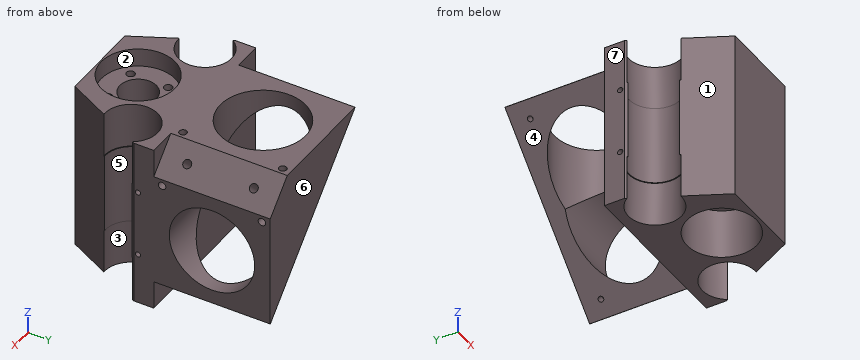
```python
from build123d import *

# Parameters (mm, degrees)
BOSS_EXTRUDE1_DEPTH        = 51
CUT_EXTRUDE1_REACH         = 53
SKETCH2_R                  = 7.75
CUT_EXTRUDE2_REACH         = 53
SKETCH6_R                  = 5.5
M3_TAPPED_HOLE2_D          = 2.5
M3_TAPPED_HOLE2_DEPTH      = 11.5
M3_TAPPED_HOLE2_TIP        = 0.751075774
SKETCH13_R                 = 10.5
CUT_EXTRUDE5_DEPTH         = 15
BOSS_EXTRUDE2_DEPTH        = 35
CUT_EXTRUDE6_REACH         = 53
SKETCH24_R                 = 12.8397
CUT_EXTRUDE7_REACH         = 53
SKETCH25_R                 = 12.8397
M2_TAPPED_HOLE1_D          = 1.6
M2_TAPPED_HOLE1_DEPTH      = 3.2
M2_TAPPED_HOLE1_TIP        = 0.480688495
M3_TAPPED_HOLE4_D          = 2.5
M3_TAPPED_HOLE4_DEPTH      = 7.5
M3_TAPPED_HOLE4_TIP        = 0.751075774
M2_TAPPED_HOLE2_AT_2_COUNT = 2
M2_TAPPED_HOLE2_AT_2_PITCH = 20
SKETCH38_R                 = 11.1
CUT_EXTRUDE8_DEPTH         = 5.5
SKETCH39_R                 = 8
CUT_EXTRUDE9_DEPTH         = 13.5
SKETCH41_R                 = 8
CUT_EXTRUDE10_DEPTH        = 13.5
F_4_40_TAPPED_HOLE1_D      = 2.2606
F_4_40_TAPPED_HOLE1_DEPTH  = 7.59
F_4_40_TAPPED_HOLE1_TIP    = 0.679152758
F_4_40_TAPPED_HOLE2_D      = 2.2606
F_4_40_TAPPED_HOLE2_DEPTH  = 7.6
F_4_40_TAPPED_HOLE2_TIP    = 0.679152758


with BuildPart() as part:
    # Sketch1 → Boss-Extrude1 (new body)
    with BuildSketch(Plane.XY):
        Polygon((-25.5, 0), (25.5, 0), (25.5, -6), (12.5, -31.5), (-12.5, -31.5), (-25.5, -6), align=None)
    extrude(amount=BOSS_EXTRUDE1_DEPTH)

    # Sketch2 → Cut-Extrude1 (cut, up to next)
    with BuildSketch(Plane.XY.offset(51), mode=Mode.PRIVATE) as cut_extrude1_sk1:
        with Locations((-18.5, -11)):
            Circle(SKETCH2_R)
    cut_extrude1_tool1 = extrude(cut_extrude1_sk1.sketch, amount=-CUT_EXTRUDE1_REACH, mode=Mode.PRIVATE) & part.part
    add(cut_extrude1_tool1.solids().sort_by_distance((-18.5, -11, 51))[0], mode=Mode.SUBTRACT)
    # Sketch2 → Cut-Extrude1 (cut, up to next)
    with BuildSketch(Plane.XY.offset(51), mode=Mode.PRIVATE) as cut_extrude1_sk2:
        with Locations((18.5, -11)):
            Circle(SKETCH2_R)
    cut_extrude1_tool2 = extrude(cut_extrude1_sk2.sketch, amount=-CUT_EXTRUDE1_REACH, mode=Mode.PRIVATE) & part.part
    add(cut_extrude1_tool2.solids().sort_by_distance((18.5, -11, 51))[0], mode=Mode.SUBTRACT)

    # Sketch6 → Cut-Extrude2 (cut, up to next)
    with BuildSketch(Plane.XY.offset(51), mode=Mode.PRIVATE) as cut_extrude2_sk1:
        with Locations((0, -20)):
            Circle(SKETCH6_R)
    cut_extrude2_tool1 = extrude(cut_extrude2_sk1.sketch, amount=-CUT_EXTRUDE2_REACH, mode=Mode.PRIVATE) & part.part
    add(cut_extrude2_tool1.solids().sort_by_distance((0, -20, 51))[0], mode=Mode.SUBTRACT)

    # M3 Tapped Hole2
    with Locations(Plane.XY.offset(51)):
        with Locations((-5.656854249, -14.343145751), (5.656854249, -25.656854249), (5.656854249, -14.343145751), (-5.656854249, -25.656854249)):
            Hole(M3_TAPPED_HOLE2_D / 2, depth=M3_TAPPED_HOLE2_DEPTH)
            with Locations((0, 0, -(M3_TAPPED_HOLE2_DEPTH + M3_TAPPED_HOLE2_TIP / 2))):  # 118° drill point
                Cone(0, M3_TAPPED_HOLE2_D / 2, M3_TAPPED_HOLE2_TIP, mode=Mode.SUBTRACT)

    # Sketch13 → Cut-Extrude5 (cut)
    with BuildSketch(Plane(origin=(0, 0, 0), x_dir=(-1, 0, 0), z_dir=(0, 0, -1))):
        with Locations((0, -20)):
            Circle(SKETCH13_R)
    extrude(amount=-CUT_EXTRUDE5_DEPTH, mode=Mode.SUBTRACT)

    # Sketch22 → Boss-Extrude2 (add)
    with BuildSketch(Plane(origin=(0, 0, 0), x_dir=(1, 0, 0), z_dir=(0, 1, 0))):
        Polygon((-16.970562748, -50.955844123), (-16.970562748, -51), (16.970562748, -51), (25.5, -42.470562748), (25.5, -8.529437252), (25.455844123, -8.529437252), align=None)
    extrude(amount=BOSS_EXTRUDE2_DEPTH)

    # Sketch24 → Cut-Extrude6 (cut, up to next)
    with BuildSketch(Plane.XY.offset(51), mode=Mode.PRIVATE) as cut_extrude6_sk1:
        with Locations((0, 17.5)):
            Circle(SKETCH24_R)
    cut_extrude6_tool1 = extrude(cut_extrude6_sk1.sketch, amount=-CUT_EXTRUDE6_REACH, mode=Mode.PRIVATE) & part.part
    add(cut_extrude6_tool1.solids().sort_by_distance((0, 17.5, 51))[0], mode=Mode.SUBTRACT)

    # Sketch25 → Cut-Extrude7 (cut, up to next)
    with BuildSketch(Plane(origin=(25.5, 0, 0), x_dir=(0, 0, -1), z_dir=(1, 0, 0)), mode=Mode.PRIVATE) as cut_extrude7_sk1:
        with Locations((-25.5, 17.5)):
            Circle(SKETCH25_R)
    cut_extrude7_tool1 = extrude(cut_extrude7_sk1.sketch, amount=-CUT_EXTRUDE7_REACH, mode=Mode.PRIVATE) & part.part
    add(cut_extrude7_tool1.solids().sort_by_distance((25.5, 17.5, 25.5))[0], mode=Mode.SUBTRACT)

    # M2 Tapped Hole1
    with Locations(Plane(origin=(16.992640687, 0, 16.992640687), x_dir=(-0.707106781, 0, 0.707106781), z_dir=(-0.707106781, 0, -0.707106781))):
        with Locations((43.03122292, 29.5), (-6.96877708, 5.5), (-6.96877708, 29.5), (43.03122292, 5.5)):
            Hole(M2_TAPPED_HOLE1_D / 2, depth=M2_TAPPED_HOLE1_DEPTH)
            with Locations((0, 0, -(M2_TAPPED_HOLE1_DEPTH + M2_TAPPED_HOLE1_TIP / 2))):  # 118° drill point
                Cone(0, M2_TAPPED_HOLE1_D / 2, M2_TAPPED_HOLE1_TIP, mode=Mode.SUBTRACT)

    # M3 Tapped Hole4
    with Locations(Plane(origin=(33.985281374, 0, 33.985281374), x_dir=(0.707106781, 0, -0.707106781), z_dir=(0.707106781, 0, 0.707106781))):
        with Locations((-18.03122292, 27.5), (-18.03122292, 7.5)):
            Hole(M3_TAPPED_HOLE4_D / 2, depth=M3_TAPPED_HOLE4_DEPTH)
            with Locations((0, 0, -(M3_TAPPED_HOLE4_DEPTH + M3_TAPPED_HOLE4_TIP / 2))):  # 118° drill point
                Cone(0, M3_TAPPED_HOLE4_D / 2, M3_TAPPED_HOLE4_TIP, mode=Mode.SUBTRACT)

    # Sketch36 → M2 Tapped Hole2 (revolve, cut)
    with BuildSketch(Plane(origin=(25.5, -4.75, 35.5), x_dir=(0, 0, -1), z_dir=(0, 1, 0))):
        Polygon((0, 0), (0, 7.680688495), (0.8, 7.2), (0.8, 0), align=None)
    m2_tapped_hole2 = revolve(axis=Axis((31.85, -4.75, 35.5), (-1, 0, 0)), mode=Mode.SUBTRACT)

    # M2 Tapped Hole2 at 2: M2 Tapped Hole2 ×2
    with Locations(*[(0, 0, -i * M2_TAPPED_HOLE2_AT_2_PITCH) for i in range(1, M2_TAPPED_HOLE2_AT_2_COUNT)]):
        add(m2_tapped_hole2, mode=Mode.SUBTRACT)

    # Mirror1: M2 Tapped Hole2 across plane
    add(m2_tapped_hole2.mirror(Plane(origin=(0, 0, 0), x_dir=(0, 0, 1), z_dir=(1, 0, 0))), mode=Mode.SUBTRACT)

    # Mirror1 copy 1 sketch → Mirror1 copy 1 (revolve, cut)
    with BuildSketch(Plane(origin=(-25.5, -4.75, 15.5), x_dir=(0, 0, -1), z_dir=(0, 1, 0))):
        Polygon((0, 0), (0, -7.680688495), (0.8, -7.2), (0.8, 0), align=None)
    revolve(axis=Axis((-31.85, -4.75, 15.5), (-1, 0, 0)), mode=Mode.SUBTRACT)

    # Sketch38 → Cut-Extrude8 (cut)
    with BuildSketch(Plane.XY.offset(51)):
        with Locations((0, -20)):
            Circle(SKETCH38_R)
    extrude(amount=-CUT_EXTRUDE8_DEPTH, mode=Mode.SUBTRACT)

    # Sketch39 → Cut-Extrude9 (cut)
    with BuildSketch(Plane(origin=(0, 0, 0), x_dir=(-1, 0, 0), z_dir=(0, 0, -1))):
        with Locations((18.5, -11)):
            Circle(SKETCH39_R)
        with Locations((-18.5, -11)):
            Circle(SKETCH39_R)
    extrude(amount=-CUT_EXTRUDE9_DEPTH, mode=Mode.SUBTRACT)

    # Sketch41 → Cut-Extrude10 (cut)
    with BuildSketch(Plane.XY.offset(51)):
        with Locations((18.5, -11)):
            Circle(SKETCH41_R)
        with Locations((-18.5, -11)):
            Circle(SKETCH41_R)
    extrude(amount=-CUT_EXTRUDE10_DEPTH, mode=Mode.SUBTRACT)

    # #4-40 Tapped Hole1
    with Locations(Plane(origin=(25.5, 0, 0), x_dir=(0, 0, -1), z_dir=(1, 0, 0))):
        with Locations((-40.5, 32.5), (-40.5, 2.5)):
            Hole(F_4_40_TAPPED_HOLE1_D / 2, depth=F_4_40_TAPPED_HOLE1_DEPTH)
            with Locations((0, 0, -(F_4_40_TAPPED_HOLE1_DEPTH + F_4_40_TAPPED_HOLE1_TIP / 2))):  # 118° drill point
                Cone(0, F_4_40_TAPPED_HOLE1_D / 2, F_4_40_TAPPED_HOLE1_TIP, mode=Mode.SUBTRACT)

    # #4-40 Tapped Hole2
    with Locations(Plane.XY.offset(51)):
        with Locations((15, 32.5), (15, 2.5)):
            Hole(F_4_40_TAPPED_HOLE2_D / 2, depth=F_4_40_TAPPED_HOLE2_DEPTH)
            with Locations((0, 0, -(F_4_40_TAPPED_HOLE2_DEPTH + F_4_40_TAPPED_HOLE2_TIP / 2))):  # 118° drill point
                Cone(0, F_4_40_TAPPED_HOLE2_D / 2, F_4_40_TAPPED_HOLE2_TIP, mode=Mode.SUBTRACT)


solid = part.part
```
Can you work these out from the model? Positions are in its coordinate system, mm. Face numbers are marked on the shaded views. A direction names the side the tool comes from. Round coordinates to 2 decimals unless told otherwise and drop trailing zeros. Loops run counter-clockwise (first coordinate to the right, second up) from the corner with the lowest first, then second, coordinate; pieces in that order, holes last. Notation, with made-up numbers: M 15,-20 L 28,-20 A9 ccw 28,-16 Z; hole C 7,3 d3. An arc over 180 degrees is marked long. Answer in a Markdown table with one row per item.
1. Thinking about a two-plate mould opening in X: for the marked faces 5, 6 and 7, which applies, pulls with the +X half, pulls with the -X half, needs draft (parallel to the pull), parting line crosses it, or undercut?
Established:
| item | result |
|---|---|
| face 5 | undercut |
| face 6 | needs draft |
| face 7 | pulls with the -X half |
2. If we section it at B-B, the plane y = 24: Please give me the cut outline in (x, z).
Established:
| item | result |
|---|---|
| outline | M -16.97,50.96 L -11.07,45.06 L -11.07,51 L -16.97,51 Z; M 11.07,36.57 L 25.5,36.57 L 25.5,42.47 L 16.97,51 L 11.07,51 Z; M 19.56,14.43 L 25.46,8.53 L 25.5,8.53 L 25.5,14.43 Z |
3. If we section it at D-D, the plane z = 6.5: Please give me the cut outline in (x, y).
Established:
| item | result |
|---|---|
| outline | M -25.5,-6 L -25.19,-6.61 A8 cw long -18.88,-18.99 L -12.5,-31.5 L 12.5,-31.5 L 18.88,-18.99 A8 cw long 25.19,-6.61 L 25.5,-6 L 25.5,0 L -25.5,0 Z; hole C 0,-20 d21 |
4. If we section it at C-C, the plane x = -18: Please give me the cut outline in (y, z).
Established:
| item | result |
|---|---|
| outline | M -20.71,0 L -18.98,0 L -18.98,13.5 L -18.73,13.5 L -18.73,37.5 L -18.98,37.5 L -18.98,51 L -20.71,51 Z; M -3.27,13.5 L -3.02,13.5 L -3.02,0 L 0,0 L 0,51 L -3.02,51 L -3.02,37.5 L -3.27,37.5 Z |
5. I'm going to push flat-ended pins straight in: pin 1 Ø1.4 at (x, y) = (15, 32.5) entering from +Z; pin 2 Ø2 at (x, y) = (5.66, -25.66) entering from -Z; pin 3 Ø12 at (y, z) = (17, 12) entering from -X; pin 4 Ø10 at (y, z) = (10.5, 26) entering from -X. Where does each tip first touch, or does it pass through?
Established:
| item | result |
|---|---|
| pin 1 | z = 43.14 |
| pin 2 | z = 15 |
| pin 3 | x = 19.79 |
| pin 4 | through |
6. If we section it at A-A, the plane z = 32: Please give me the cut outline in (x, y), plus the area to 3 significant figures.
Established:
| item | result |
|---|---|
| outline | M -25.5,-6 L -25.06,-6.87 A7.75 cw long -19.01,-18.73 L -12.5,-31.5 L 12.5,-31.5 L 19.01,-18.73 A7.75 cw long 25.06,-6.87 L 25.5,-6 L 25.5,6.43 L 6.5,6.43 A12.84 cw 1.99,4.81 L 1.99,0 L -25.5,0 Z; M 1.99,30.19 A12.84 cw 6.5,28.57 L 25.5,28.57 L 25.5,35 L 1.99,35 Z; hole C 0,-20 d11 |
| area | 1,170 mm² |
7. Please list where these lines run through material, in increasing order: line 1 (Z direction, x = -24.2, y = -4.75); line 2 (Y direction, x = 17, z = 23.5); line 3 (Y direction, x = 14.5, z = 25.5). Write a range as from..to.
Established:
| item | result |
|---|---|
| line 1 | 0..14.7, 16.3..34.7, 36.3..51 |
| line 2 | -22.67..-18.6, -3.4..4.82, 30.18..35 |
| line 3 | -27.58..-17.64, -4.36..4.66, 30.34..35 |
8. On a 3-axis mill with a long thin cutter (end or side, diameter ignored), from which of +Z, -Z, +X, -X, +Y, -Y can I reach the whole of each face in a straight line? I mean the marked faces 1, 2, 3 and 4. Say none if no direction works.
Established:
| item | result |
|---|---|
| face 1 | +Z, -Z, -X, -Y |
| face 2 | +Z |
| face 3 | -Z |
| face 4 | -Z, -X, +Y |
